The model under review builds one solid part; all positions refer to its coordinate system, in mm. Face numbers are marked on the shaded views. A direction names the side the tool comes from. Round coordinates to 2 decimals unless told otherwise and drop trailing zeros. Loops run counter-clockwise (first coordinate to the right, second up) from the corner with the lowest first, then second, coordinate; pieces in that order, holes last. Notation, with made-up numbers: M 23.25,68 L 34.25,68 A19 ccw 34.25,94 Z; hole C 3.25,41.5 d1. An arc over 180 degrees is marked long. Answer in a Markdown table with one row per item. Add a question column.
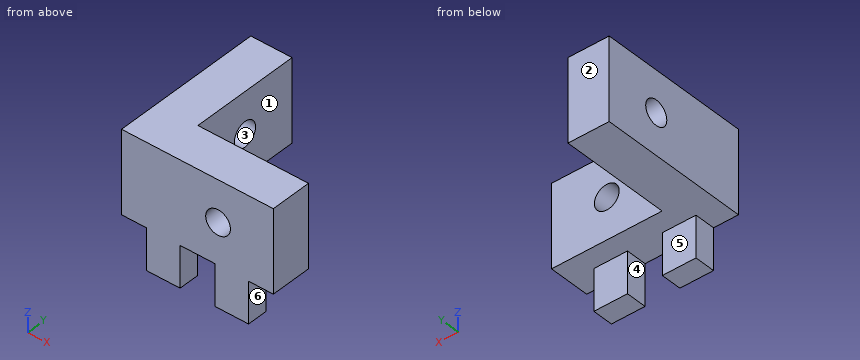
from build123d import *

# Parameters (mm, degrees)
BOSS_EXTRUDE1_DEPTH = 10
CUT_EXTRUDE1_REACH  = 22.962
SKETCH2_R           = 1.5
CUT_EXTRUDE2_REACH  = 22.893
SKETCH3_R           = 1.5
SKETCH4_W           = 4.077350098
SKETCH4_H           = 5
SKETCH4_W_2         = 4.08
BOSS_EXTRUDE2_DEPTH = 2.5


with BuildPart() as part:
    # Sketch1 → Boss-Extrude1 (new body)
    with BuildSketch(Plane.XY):
        Polygon((-0.757575758, 12.528787879), (-5.757575758, 12.528787879), (-5.757575758, -5.871212121), (12.642424242, -5.871212121), (12.642424242, -0.871212121), (-0.757575758, -0.871212121), align=None)
    extrude(amount=BOSS_EXTRUDE1_DEPTH)

    # Sketch2 → Cut-Extrude1 (cut, up to next)
    with BuildSketch(Plane(origin=(0, -0.871212121, 0), x_dir=(1, 0, 0), z_dir=(0, 1, 0)), mode=Mode.PRIVATE) as cut_extrude1_sk1:
        with Locations(Location((5.942424242, -5, 0), (0, 0, 180))):
            Circle(SKETCH2_R)
    cut_extrude1_tool1 = extrude(cut_extrude1_sk1.sketch, amount=-CUT_EXTRUDE1_REACH, mode=Mode.PRIVATE) & part.part
    add(cut_extrude1_tool1.solids().sort_by_distance((5.942424, -0.871212, 5))[0], mode=Mode.SUBTRACT)

    # Sketch3 → Cut-Extrude2 (cut, up to next)
    with BuildSketch(Plane(origin=(-0.757575758, 0, 0), x_dir=(0, 0, -1), z_dir=(1, 0, 0)), mode=Mode.PRIVATE) as cut_extrude2_sk1:
        with Locations((-5, 5.828787879)):
            Circle(SKETCH3_R)
    cut_extrude2_tool1 = extrude(cut_extrude2_sk1.sketch, amount=-CUT_EXTRUDE2_REACH, mode=Mode.PRIVATE) & part.part
    add(cut_extrude2_tool1.solids().sort_by_distance((-0.757576, 5.828788, 5))[0], mode=Mode.SUBTRACT)

    # Sketch4 → Boss-Extrude2 (add)
    with BuildSketch(Plane.XZ.offset(5.871212121)):
        with Locations((7.603749193, -2.5)):
            Rectangle(SKETCH4_W, SKETCH4_H)
        with Locations((-0.697575758, -2.5)):
            Rectangle(SKETCH4_W_2, SKETCH4_H)
    extrude(amount=-BOSS_EXTRUDE2_DEPTH)


solid = part.part
1. To check wall thickness, follow probe 1 along X at (y, z) = (9.75, 3.5); probe 2 along Y at (x, z) = (9.75, 1.75); probe 3 along Z at (x, y) = (-3, 3.5). State the ranges of each line that lie inside material, in increasing order.
2. Take a section at B-B, the plane x = 5. State the section outline as (y, z) points, and give its area (3 significant figures).
3. Machinability: for the marked faces 4, 5 and 6, which of the approach directions +Z, -Z, +X, -X, +Y, -Y give a long, thin tool a straight path to every point of the face, cutting with its end or side? Answer none if there is none.
4. Take a section at C-C, the plane x = 8.5. State the section outline as (y, z) points, and give its area (3 significant figures).
5. For pin 1 Ø2 at (y, z) = (-4.5, -2) entering from -X; pin 2 Ø3 at (x, z) = (0.5, -2.5) entering from +Y; pin 3 Ø5 at (y, z) = (8.5, 8.5) entering from +X, all flat-tipped, find the tip position at first contact; note any pin that passes through.
6. Take a section at D-D, the plane y = 8. State the section outline as (x, z) points.
7. Take a section at A-A, the plane z = 5. State the section outline as (x, y) points, and give its area (3 significant figures).
8. Mouldability with a two-part tool opening along Y and no side actions: class the marked faces 1, 2 and 3 as released by +Y, released by -Y, zero draft, split by the parting line, or undercut.
Check sheet entries:
| question | item | result |
|---|---|---|
| 1 | probe 1 | x = -5.76 to -0.76 |
| 1 | probe 2 | y = -5.87 to -0.87 |
| 1 | probe 3 | z = 0 to 10 |
| 2 | outline | M -5.87,0 L -0.87,0 L -0.87,3.83 L -5.87,3.83 Z; M -5.87,6.17 L -0.87,6.17 L -0.87,10 L -5.87,10 Z |
| 2 | area | 38.3 mm^2 |
| 3 | face 4 | -Z, +Y, -Y |
| 3 | face 5 | -Z, +X, -X, +Y |
| 3 | face 6 | -Z, +X, +Y, -Y |
| 4 | outline | M -5.87,-5 L -3.37,-5 L -3.37,0 L -0.87,0 L -0.87,10 L -5.87,10 Z |
| 4 | area | 62.5 mm^2 |
| 5 | pin 1 | stops at x = -2.74 |
| 5 | pin 2 | stops at y = -3.37 |
| 5 | pin 3 | stops at x = -0.76 |
| 6 | outline | M -5.76,0 L -0.76,0 L -0.76,10 L -5.76,10 Z |
| 7 | outline | M -5.76,-5.87 L 4.44,-5.87 L 4.44,-0.87 L -0.76,-0.87 L -0.76,4.33 L -5.76,4.33 Z; M -5.76,7.33 L -0.76,7.33 L -0.76,12.53 L -5.76,12.53 Z; M 7.44,-5.87 L 12.64,-5.87 L 12.64,-0.87 L 7.44,-0.87 Z |
| 7 | area | 129 mm^2 |
| 8 | face 1 | zero draft |
| 8 | face 2 | released by +Y |
| 8 | face 3 | undercut |
